Could you check a few things on this model? Use its own coordinates, in mm. A direction names the side the tool comes from. Coordinates: 2 decimals unless noted, no trailing zeros. Loops run counter-clockwise (first coordinate to the right, second up) from the corner with the lowest first, then second, coordinate; pieces in that order, holes last. Notation, with made-up numbers: (73, -10) -> (132, -10) arc R8 cw to (132, -6) -> close; hole circle Ø1 at (3.25, 4). An arc over 180 degrees is marked (long way). One line per question, with ' | ' between items.
from build123d import *

# Parameters (mm, degrees)
SKETCH_1_R          = 16.5
EXTRUDE_1_DEPTH     = 2
SKETCH_2_R          = 8.5
EXTRUDE_2_DEPTH     = 12
SKETCH_3_R          = 5.4
CUT_EXTRUDE_1_DEPTH = 29
SKETCH_4_R          = 1.6
CUT_EXTRUDE_2_DEPTH = 29
SKETCH_7_R          = 1.5
CUT_EXTRUDE_3_DEPTH = 12


with BuildPart() as part:
    # Sketch 1 → Extrude 1 (new body)
    with BuildSketch(Plane.XY):
        Circle(SKETCH_1_R)
    extrude(amount=EXTRUDE_1_DEPTH)

    # Sketch 2 → Extrude 2 (add)
    with BuildSketch(Plane.XY.offset(2)):
        Circle(SKETCH_2_R)
    extrude(amount=EXTRUDE_2_DEPTH)

    # Sketch 3 → Cut-Extrude 1 (cut)
    with BuildSketch(Plane.XY.offset(14)):
        Circle(SKETCH_3_R)
    extrude(amount=-CUT_EXTRUDE_1_DEPTH, mode=Mode.SUBTRACT)

    # Sketch 4 → Cut-Extrude 2 (cut)
    with BuildSketch(Plane(origin=(0, 0, 0), x_dir=(-1, 0, 0), z_dir=(0, 0, -1))):
        with Locations((0, 12)):
            Circle(SKETCH_4_R)
        with Locations((10.392304845, -6)):
            Circle(SKETCH_4_R)
        with Locations((-10.392304845, -6)):
            Circle(SKETCH_4_R)
    extrude(amount=-CUT_EXTRUDE_2_DEPTH, mode=Mode.SUBTRACT)

    # Sketch 7 → Cut-Extrude 3 (cut)
    with BuildSketch(Plane(origin=(0, 0, 0), x_dir=(1, 0, 0), z_dir=(0, 1, 0))):
        with Locations(Location((0, -9.5, 0), (0, 0, 270))):
            Circle(SKETCH_7_R)
    extrude(amount=-CUT_EXTRUDE_3_DEPTH, mode=Mode.SUBTRACT)


solid = part.part
1) If we section it at A-A on x = 0: Please give me the cut outline in (y, z).
Data:
outline: (-16.5, 0) -> (-5.4, 0) -> (-5.4, 8) -> (-8.5, 8) -> (-8.5, 2) -> (-16.5, 2) -> close; (-8.5, 11) -> (-5.4, 11) -> (-5.4, 14) -> (-8.5, 14) -> close; (5.4, 0) -> (10.4, 0) -> (10.4, 2) -> (8.5, 2) -> (8.5, 14) -> (5.4, 14) -> close; (13.6, 0) -> (16.5, 0) -> (16.5, 2) -> (13.6, 2) -> close
2) On a 3-axis mill with a long thin cutter (end or side, diameter ignored), from which of +Z, -Z, +X, -X, +Y, -Y can I reach the whole of each face in a straight line? I mean faces 5 (the face through (-4, 4, 0)), 6 (the face through (0, -7, 8)), 7 (the face through (4.57, 7.167, 7.916)). Say none if no direction works.
Data:
face 5: -Z, +X, -X, +Y, -Y | face 6: -Y | face 7: +Z
3) If we section it at B-B on y = 0: Please give me the cut outline in (x, z).
Data:
outline: (-16.5, 0) -> (-5.4, 0) -> (-5.4, 14) -> (-8.5, 14) -> (-8.5, 2) -> (-16.5, 2) -> close; (5.4, 0) -> (16.5, 0) -> (16.5, 2) -> (8.5, 2) -> (8.5, 14) -> (5.4, 14) -> close
4) If we section it at D-D on x = 4: Please give me the cut outline in (y, z), and give its area (3 significant figures).
Data:
outline: (-16.01, 0) -> (-3.63, 0) -> (-3.63, 14) -> (-7.5, 14) -> (-7.5, 2) -> (-16.01, 2) -> close; (3.63, 0) -> (16.01, 0) -> (16.01, 2) -> (7.5, 2) -> (7.5, 14) -> (3.63, 14) -> close | area: 142 mm²
5) I need wall thicknesses on line 1 along Z through (x, y) = (-11.5, 1); line 2 along X through (y, z) = (-3, 5.25); line 3 along Y through (x, z) = (-4, 12.5). Which ranges of each line are inside material? Lowest first, please. Write a range as from..to.
Data:
line 1: 0..2 | line 2: -7.95..-4.49, 4.49..7.95 | line 3: -7.5..-3.63, 3.63..7.5
6) I'm going to push flat-ended pins straight in: pin 1 Ø5 at (y, z) = (7, 11.5) entering from -X; pin 2 Ø3.5 at (x, y) = (0, 12) entering from +Z; pin 3 Ø3 at (y, z) = (10.5, 11) entering from -X; pin 4 Ø8 at (x, z) = (-8, 12) entering from +Y. Where does each tip first touch, or does it pass through?
Data:
pin 1: x = -7.21 | pin 2: z = 2 | pin 3: through | pin 4: y = 7.5
7) We'd pull the mould along Y, two halves only. Please class faces 1 (the face through (-4, 8, 2)), 2 (the face through (0.208, 13.586, 0.986)), 3 (the face through (15.24, -6.32, 0.99)), 4 (the face through (11.662, -6.974, 0.986)): pulls with the +Y half, pulls with the -Y half, needs draft (parallel to the pull), parting line crosses it, or undercut.
Data:
face 1: needs draft | face 2: undercut | face 3: parting line crosses it | face 4: undercut
8) If we section it at C-C on y = -6: Please give me the cut outline in (x, z), and give its area (3 significant figures).
Data:
outline: (-15.37, 0) -> (-11.99, 0) -> (-11.99, 2) -> (-15.37, 2) -> close; (-8.79, 0) -> (8.79, 0) -> (8.79, 2) -> (6.02, 2) -> (6.02, 14) -> (-6.02, 14) -> (-6.02, 2) -> (-8.79, 2) -> close; (11.99, 0) -> (15.37, 0) -> (15.37, 2) -> (11.99, 2) -> close; hole circle Ø3 at (0, 9.5) | area: 186 mm²
